Verification items for the finished model (mm, model axes). A direction names the side the tool comes from. Round coordinates to 2 decimals unless told otherwise and drop trailing zeros. Write each loop counter-clockwise with the first axis right and the second up, starting at its lowest first coordinate (ties: lowest second). Pieces come first, ordered by that corner, then holes. Notation, with made-up numbers: M -20.5,-14.75 L 38.5,-14.75 A11 cw 38.5,-8.75 Z; hole C 51,-28.5 d2. An arc over 180 degrees is marked long. Write each question's results on one line, items separated by ' | '.
from build123d import *

# Parameters (mm, degrees)
SKETCH1_W           = 73
SKETCH1_H           = 140
BOSS_EXTRUDE1_DEPTH = 16
SKETCH2_W           = 67.5
SKETCH2_H           = 135
CUT_EXTRUDE1_DEPTH  = 13
SKETCH3_W           = 14.2
SKETCH3_H           = 6.45
SKETCH3_W_2         = 10.9
SKETCH3_H_2         = 4.8
CUT_EXTRUDE2_DEPTH  = 2.5
FILLET1_R           = 3
SKETCH4_W           = 10.2
SKETCH4_H           = 5.5
CUT_EXTRUDE3_DEPTH  = 2.75
FILLET2_R           = 1
FILLET3_R           = 1
FILLET4_R           = 2
CHAMFER1_SIZE       = 1
SKETCH6_W           = 92.196914974
SKETCH6_H           = 18.56524909
CUT_EXTRUDE4_DEPTH  = 159.697826072


with BuildPart() as part:
    # Sketch1 → Boss-Extrude1 (new body)
    with BuildSketch(Plane(origin=(0, 0, 0), x_dir=(1, 0, 0), z_dir=(0, 1, 0))):
        with Locations((36.5, 70)):
            Rectangle(SKETCH1_W, SKETCH1_H)
    extrude(amount=BOSS_EXTRUDE1_DEPTH)

    # Sketch2 → Cut-Extrude1 (cut)
    with BuildSketch(Plane(origin=(0, 16, 0), x_dir=(1, 0, 0), z_dir=(0, 1, 0))):
        with Locations((36.5, 70)):
            Rectangle(SKETCH2_W, SKETCH2_H)
    extrude(amount=-CUT_EXTRUDE1_DEPTH, mode=Mode.SUBTRACT)

    # Sketch3 → Cut-Extrude2 (cut)
    with BuildSketch(Plane.XY):
        with Locations((20.05, 11.125)):
            Rectangle(SKETCH3_W, SKETCH3_H)
        with Locations((36.6, 11.95)):
            Rectangle(SKETCH3_W_2, SKETCH3_H_2)
        with Locations((53.15, 11.125)):
            Rectangle(SKETCH3_W, SKETCH3_H)
    extrude(amount=-CUT_EXTRUDE2_DEPTH, mode=Mode.SUBTRACT)

    # Fillet1
    fillet1_edges = [part.edges().sort_by_distance(p)[0] for p in [
        (0, 8, -140),
        (73, 8, -140),
        (73, 8, 0),
        (0, 8, 0),
    ]]
    fillet(fillet1_edges, radius=FILLET1_R)

    # Sketch4 → Cut-Extrude3 (cut)
    with BuildSketch(Plane(origin=(73, 0, 0), x_dir=(0, 0, -1), z_dir=(1, 0, 0))):
        with Locations((17.7, 10.6)):
            Rectangle(SKETCH4_W, SKETCH4_H)
    extrude(amount=-CUT_EXTRUDE3_DEPTH, mode=Mode.SUBTRACT)

    # Fillet2
    fillet2_edges = [part.edges().sort_by_distance(p)[0] for p in [
        (27.15, 14.35, -1.25),
        (27.15, 7.9, -1.25),
        (12.95, 7.9, -1.25),
        (12.95, 14.35, -1.25),
        (31.15, 9.55, -1.25),
        (31.15, 14.35, -1.25),
        (42.05, 14.35, -1.25),
        (42.05, 9.55, -1.25),
        (60.25, 7.9, -1.25),
        (46.05, 7.9, -1.25),
        (46.05, 14.35, -1.25),
        (60.25, 14.35, -1.25),
    ]]
    fillet(fillet2_edges, radius=FILLET2_R)

    # Fillet3
    fillet3_edges = [part.edges().sort_by_distance(p)[0] for p in [
        (0, 16, -70),
        (36.5, 16, -140),
        (36.5, 16, 0),
        (73, 16, -70),
        (0.878679656, 16, -0.878679656),
        (72.121320344, 16, -0.878679656),
        (72.121320344, 16, -139.121320344),
        (0.878679656, 16, -139.121320344),
    ]]
    fillet(fillet3_edges, radius=FILLET3_R)

    # Fillet4
    fillet4_edges = [part.edges().sort_by_distance(p)[0] for p in [
        (2.75, 9.5, -2.5),
        (2.75, 9.5, -137.5),
        (70.25, 9.5, -137.5),
        (70.25, 9.5, -2.5),
    ]]
    fillet(fillet4_edges, radius=FILLET4_R)

    # Chamfer1
    chamfer1_edges = [part.edges().sort_by_distance(p)[0] for p in [
        (70.25, 16, -70),
        (36.5, 16, -2.5),
        (36.5, 16, -137.5),
        (2.75, 16, -70),
        (69.664213562, 16, -3.085786438),
        (69.664213562, 16, -136.914213562),
        (3.335786438, 16, -136.914213562),
        (3.335786438, 16, -3.085786438),
    ]]
    chamfer(chamfer1_edges, length=CHAMFER1_SIZE)

    # Sketch6 → Cut-Extrude4 (cut, through all)
    with BuildSketch(Plane.XY):
        with Locations((35.320005354, 20.832624545)):
            Rectangle(SKETCH6_W, SKETCH6_H)
    extrude(amount=-CUT_EXTRUDE4_DEPTH, mode=Mode.SUBTRACT)


solid = part.part
1) Access from +Z, -Z, +X, -X, +Y, -Y to the whole of each face (thin tool, end or side, straight path). Record for faces 1 (the flat face through (72, 7.85, -18)), 2 (the flat face through (70.25, 7, -69)), 3 (the flat face through (27.15, 10, -1)), 4 (the flat face through (44, 11.55, -1)).
Calculated:
face 1: +X, +Y | face 2: +Y | face 3: +Z, +Y | face 4: +Z, -Z, +X, -X, +Y
2) Draft check along X on faces 5 (the flat face through (36, 6, -2.5)), 6 (the cylindrical face through (0.86, 5.86, -0.9)), 7 (the cylindrical face through (72.1, 5.86, -0.86)). Enter one of: pulls with the +X half, pulls with the -X half, needs draft (parallel to the pull), parting line crosses it, or undercut.
Calculated:
face 5: undercut | face 6: pulls with the -X half | face 7: pulls with the +X half
3) Sectioned sample at A-A, the plane z = -102. Record the cut outline in (x, y), and give its area (3 significant figures).
Calculated:
outline: M 0,0 L 73,0 L 73,11.55 L 70.25,11.55 L 70.25,3 L 2.75,3 L 2.75,11.55 L 0,11.55 Z | area: 266 mm²
4) Sectioned sample at B-B, the plane x = 34.5. Record the cut outline in (y, z).
Calculated:
outline: M 0,-140 L 11.55,-140 L 11.55,-137.5 L 3,-137.5 L 3,-2.5 L 9.55,-2.5 L 9.55,0 L 0,0 Z
5) Sectioned sample at C-C, the plane y = 6.5. Record the cut outline in (x, z).
Calculated:
outline: M 0,-137 A3 ccw 3,-140 L 70,-140 A3 ccw 73,-137 L 73,-3 A3 ccw 70,0 L 3,0 A3 ccw 0,-3 Z; hole M 2.75,-135.5 A2 ccw 4.75,-137.5 L 68.25,-137.5 A2 ccw 70.25,-135.5 L 70.25,-4.5 A2 ccw 68.25,-2.5 L 4.75,-2.5 A2 ccw 2.75,-4.5 Z
6) Depth check by flat-ended pin: P1, Ø0.5, axis at y = 11, z = -1, coming from the +X side; P2, Ø0.8, axis at x = 71, y = 10, coming from the +Z side; P3, Ø0.8, axis at x = 34.5, z = -1, coming from the +Y side. Enter the tip coordinate at first touch or a pass-through.
Calculated:
P1: stops at x = 72.44 | P2: stops at z = -0.06 | P3: stops at y = 9.55
7) Material ranges on line 1 (X direction, y = 10.75, z = -102); line 2 (Z direction, x = 62.5, y = 3.75); line 3 (Y direction, x = 42, z = -55), recorded low to high. Write a range as [from, to].
Calculated:
line 1: x = [0, 2.75], [70.25, 73] | line 2: z = [-140, -137.5], [-2.5, 0] | line 3: y = [0, 3]
